Here's how the part is built. I have some questions about the finished solid (model axes, mm). A direction names the side the tool comes from. Coordinates: 2 decimals unless noted, no trailing zeros. Order: outer loops, then holes, each group sorted by start corner. A loop starts at its lowest first (then second) coordinate and runs counter-clockwise, first axis right, second up. Notation, with made-up numbers: M 30,41.25 L 67,41.25 A23 ccw 67,69.25 Z; hole C 0.5,14 d9. An arc over 180 degrees is marked long. Answer as CSV lines item,"result". Start each with the question number.
Autodesk Fusion 360 part; units mm, degrees
sketch "Boceto1" plane through (0, 0, 0) normal (0, 0, 1) x (1, 0, 0)
  line L0 (0, 10) -> (-9.5106, 3.0902)
  line L1 (-9.5106, 3.0902) -> (-5.8779, -8.0902)
  line L2 (-5.8779, -8.0902) -> (5.8779, -8.0902)
  line L3 (5.8779, -8.0902) -> (9.5106, 3.0902)
  line L4 (9.5106, 3.0902) -> (0, 10)
  line L5 (-9.0281, 2.7396) -> (-5.6882, -7.738)
  line L6 (-5.3954, -7.7396) -> (5.4788, -7.8003)
  line L7 (5.6936, -7.523) -> (9.1501, 2.9168)
  line L8 (8.9142, 3.0902) -> (0.1524, 9.5309)
  line L9 (-0.1843, 9.4328) -> (-9.0173, 3.0902)
  line L10 (-9.0173, 3.0902) -> (-2.2451, 3.0902)
  line L11 (2.2451, 3.0902) -> (8.9142, 3.0902)
  line L12 (-9.0281, 2.7396) -> (-3.6327, -1.1803)
  line L13 (0, -3.8197) -> (5.4788, -7.8003)
  line L14 (9.1115, 2.8003) -> (3.6327, -1.1803)
  line L15 (0, -3.8197) -> (-5.3954, -7.7396)
  line L16 (-0.1843, 9.4328) -> (-2.2451, 3.0902)
  line L17 (-3.6327, -1.1803) -> (-5.7254, -7.6211)
  line L18 (0.1524, 9.5309) -> (2.2451, 3.0902)
  line L19 (3.6327, -1.1803) -> (5.6936, -7.523)
extrude "Extruir1" add sketch "Boceto1" along normal blind 0.5 contours L5 L12 L17 | L6 L13 L15 | L7 L14 L19 | L8 L11 L18 | L9 L10 L16 makes body 1 at (0.0278, -6.4532, 0) makes body 2 at (-6.1287, -2.0206, 0) makes body 3 at (6.1459, -1.9677, 0) makes body 4 at (-3.8156, 5.2044, 0) makes body 5 at (3.7706, 5.2371, 0)
extrude "Extruir2" add sketch "Boceto1" along normal blind 1 bodies 1 2 3 4 5
1) Which directions (+Z, -Z, +X, -X, +Y, -Y) give clear straight access to the entire face, cutting with the end or side of a thin tool? Please do faces 1 (the face through (6, -2, 0.5)), 2 (the face through (-4.689, 6.593, 0.493)).
2) Suppose I cut it at D-D on x = 5. Please give me the cut outline in (y, z), plus the area to 3 significant figures.
3) I need wall thicknesses on line 1 (Y direction, x = -3, z = 0.85); line 2 (X direction, y = 4.25, z = 0.6); line 3 (X direction, y = 2.5, z = 0.75). Which ranges of each line are inside material? Lowest first, please. Write a range as [from, to].
4) Suppose I cut it at A-A on x = 7.5. Please give me the cut outline in (y, z), plus the area to 3 significant figures.
5) Suppose I cut it at B-B on z = 0.3. Please give me the cut outline in (x, y).
6) Suppose I cut it at C-C on y = -1.75. Please give me the cut outline in (x, z), plus the area to 3 significant figures.
7) Will these pins go through, and if not, where does the flat tip stop? pin 1 Ø4.5 at (x, y) = (-5.5, -4.5) entering from +Z; pin 2 Ø1.9 at (x, y) = (3.5, 5) entering from +Z.
8) If we mould it in two halves opening along Y, with no side actions, what happens to faces 3 (the face through (0, -1, 0)), 4 (the face through (4.82, 6.5, 0.49)), 5 (the face through (7.67, -2.58, 0.49)), 6 (the face through (6.41, 0.84, 0.75))? For each: released by +Y, released by -Y, zero draft, split by the parting line, or undercut.
Output:
1,face 1,"+Z"
1,face 2,"+Z, -Z, -X, +Y"
2,outline,"M -8.09,0 L 6.37,0 L 6.37,1 L 5.97,1 L 5.97,0.5 L 3.09,0.5 L 3.09,1 L -0.19,1 L -0.19,0.5 L -5.39,0.5 L -5.39,1 L -7.45,1 L -7.45,0.5 L -7.8,0.5 L -7.8,1 L -8.09,1 Z"
2,area,"10.2 mm²"
3,line 1,"[-8.09, -7.75], [-6, 3.09], [7.41, 7.82]"
3,line 2,"[-7.91, -7.4], [-1.87, 1.87], [7.34, 7.91]"
3,line 3,"[-9.32, -8.95], [-8.7, 8.7], [9.01, 9.32]"
4,outline,"M -3.1,0 L 4.55,0 L 4.55,1 L 4.13,1 L 4.13,0.5 L 3.09,0.5 L 3.09,1 L 1.63,1 L 1.63,0.5 L -2.07,0.5 L -2.07,1 L -3.1,1 Z"
4,area,"5.28 mm²"
5,outline,"M -9.51,3.09 L -5.88,-8.09 L 5.88,-8.09 L 9.51,3.09 L 0,10 Z"
6,outline,"M -7.94,0 L 7.94,0 L 7.94,1 L 7.6,1 L 7.6,0.5 L 3.82,0.5 L 3.82,1 L -3.82,1 L -3.82,0.5 L -7.6,0.5 L -7.6,1 L -7.94,1 Z"
6,area,"12.1 mm²"
7,pin 1,"z = 1"
7,pin 2,"z = 0.5"
8,face 3,"zero draft"
8,face 4,"released by +Y"
8,face 5,"released by -Y"
8,face 6,"undercut"
